Read the model definition and answer for the solid it produces. Units are mm, in the model's axes. Give positions to 0.01 mm unless a question says otherwise; leave off trailing zeros. Write each loop counter-clockwise with the first axis right and the second up, starting at its lowest first coordinate (ties: lowest second). Pieces come first, ordered by that corner, then holes. Notation, with made-up numbers: (70.25, 17) -> (121.25, 17) arc R10 cw to (121.25, 22) -> close; hole circle Ø3 at (28, 39). An arc over 180 degrees is marked (long way). Answer as CSV lines item,"result". Start each with the question number.
1. The part is cut by section A-A, the plane x = 0.85. Determine the outline of the cut face in (y, z), and give its area (3 significant figures).
2. Find the intervals of material crossed by line 1 (X direction, y = 16, z = -0.5); line 2 (Y direction, x = 0.1, z = -1.5); line 3 (Z direction, x = 0.15, y = 13), in increasing order.
3. Given pin 1 (1 mm diameter, centred on x = 1.5, z = -3.5, fed in from +Y), flat-ended and moving along its own axis, determine where the tip first touches the part or whether it passes through.
from build123d import *

# Parameters (mm, degrees)
BOSS_EXTRUDE1_DEPTH      = 5
BOSS_EXTRUDE1_DEPTH_BACK = 5
SKETCH1_W                = 4
SKETCH1_H                = 50
CUT_EXTRUDE1_DEPTH       = 60
FILLET2_R                = 2
FILLET3_R                = 0.5


with BuildPart() as part:
    # Sketch1 → Boss-Extrude1 (new, two sides: drawn at the far end of the back side and taken through both)
    with BuildSketch(Plane.XY.offset(-BOSS_EXTRUDE1_DEPTH_BACK)):
        Rectangle(SKETCH1_W, SKETCH1_H)
    extrude(amount=BOSS_EXTRUDE1_DEPTH + BOSS_EXTRUDE1_DEPTH_BACK)

    # Sketch2 → Cut-Extrude1 (cut)
    with BuildSketch(Plane(origin=(0, 25, 0), x_dir=(1, 0, 0), z_dir=(0, 1, 0))):
        with BuildLine():
            Line((-2, 5), (-2, 0))
            Line((-2, 0), (-1, 0))
            add(Edge.make_bspline(
                [(-2, 5), (-1, 2.5), (-1, 0)],
                knots=[0, 0, 0, 0.5, 0.5, 0.5], degree=2))
        make_face()
        with BuildLine():
            Line((-1, 0), (-2, 0))
            Line((-2, 0), (-2, -5))
            add(Edge.make_bspline(
                [(-1, 0), (-1, -2.5), (-2, -5)],
                knots=[0.5, 0.5, 0.5, 1, 1, 1], degree=2))
        make_face()
    extrude(amount=-CUT_EXTRUDE1_DEPTH, mode=Mode.SUBTRACT)

    # Fillet2
    fillet2_edges = [part.edges().sort_by_distance(p)[0] for p in [
        (2, 0, 5),
        (2, 0, -5),
        (2, 25, 0),
    ]]
    fillet(fillet2_edges, radius=FILLET2_R)

    # Fillet3
    fillet3_edges = [part.edges().sort_by_distance(p)[0] for p in [
        (-2, 0, -5),
        (-2, 0, 5),
    ]]
    fillet(fillet3_edges, radius=FILLET3_R)


solid = part.part
Results found:
1,outline,"(-25, -4.81) -> (24.81, -4.81) -> (24.81, 4.81) -> (-25, 4.81) -> close"
1,area,"479 mm²"
2,line 1,"x = -1.01 to 2"
2,line 2,"y = -25 to 25"
2,line 3,"z = -4.99 to 4.99"
3,pin 1,"stops at y = 24.73"
